Input: part model. Units: mm. Frame: model coordinates. Face numbers are marked on the shaded views. Coordinates: 2 decimals unless noted, no trailing zeros. Loops run counter-clockwise (first coordinate to the right, second up) from the corner with the lowest first, then second, coordinate; pieces in that order, holes last. Notation, with made-up numbers: M 30.5,72 L 65.5,72 A29 cw 65.5,95 Z; hole C -24.5,64 d3. An arc over 180 degrees is marked long. Use a Markdown table: item, result. Add a question column.
1. Draft query along Y for the marked faces 1 and 2. Return one class per face: +Y half, -Y half, draft (parallel to the pull), parting line (faces both ways), or undercut.
2. Line query: L1, parallel to X at y = 10, z = 0; L2, parallel to X at y = 9, z = 179; L3, parallel to Z at x = -277, y = 6.5. Output: solid intervals per line, ascending. Write a range as [from, to].
3. Pin query (flat end, axial travel): pin 1 (12 mm diameter, centred on x = 104.5, y = 2.5, fed in from +Z); pin 2 (1 mm diameter, centred on y = 4.5, z = -58.5, fed in from +X); pin 3 (12 mm diameter, centred on x = -34.5, y = 6.5, fed in from +Z). Return the tip coordinate at first contact, or that it passes through.
4. Section A-A on x = 0. Output: boundary loops of the cut face in (y, z), then the cut area to 3 significant figures.
5. Section B-B on z = 0. Output: boundary loops of the cut face in (x, y), then the cut area to 3 significant figures.
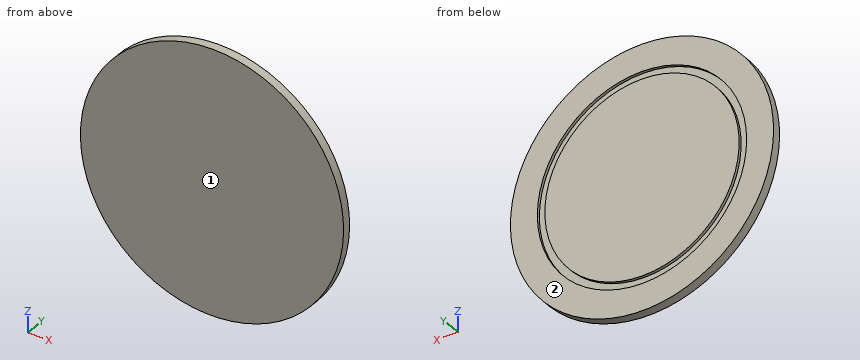
```python
from build123d import *

# Parameters (mm, degrees)
SKETCH1_R           = 440
BOSS_EXTRUDE1_DEPTH = 15
SKETCH2_R           = 350
SKETCH2_R_2         = 325
CUT_EXTRUDE1_DEPTH  = 10


with BuildPart() as part:
    # Sketch1 → Boss-Extrude1 (new, symmetric)
    with BuildSketch(Plane(origin=(0, 0, 0), x_dir=(1, 0, 0), z_dir=(0, 1, 0))):
        with Locations(Location((0, 0, 0), (0, 0, 270))):
            Circle(SKETCH1_R)
    extrude(amount=BOSS_EXTRUDE1_DEPTH, both=True)

    # Sketch2 → Cut-Extrude1 (cut)
    with BuildSketch(Plane(origin=(0, 15, 0), x_dir=(1, 0, 0), z_dir=(0, 1, 0))):
        with Locations(Location((0, 0, 0), (0, 0, 270))):
            Circle(SKETCH2_R)
        with Locations(Location((0, 0, 0), (0, 0, 270))):
            Circle(SKETCH2_R_2, mode=Mode.SUBTRACT)
    extrude(amount=-CUT_EXTRUDE1_DEPTH, mode=Mode.SUBTRACT)


solid = part.part
```
Answers below:
| question | item | result |
|---|---|---|
| 1 | face 1 | -Y half |
| 1 | face 2 | +Y half |
| 2 | L1 | x = [-440, -350], [-325, 325], [350, 440] |
| 2 | L2 | x = [-401.94, -300.76], [-271.26, 271.26], [300.76, 401.94] |
| 2 | L3 | z = [-341.86, -213.94], [-169.99, 169.99], [213.94, 341.86] |
| 3 | pin 1 | stops at z = 428.83 |
| 3 | pin 2 | stops at x = 436.16 |
| 3 | pin 3 | stops at z = 439.08 |
| 4 | outline | M -15,-440 L 15,-440 L 15,-350 L 5,-350 L 5,-325 L 15,-325 L 15,325 L 5,325 L 5,350 L 15,350 L 15,440 L -15,440 Z |
| 4 | area | 25,900 mm² |
| 5 | outline | M -440,-15 L 440,-15 L 440,15 L 350,15 L 350,5 L 325,5 L 325,15 L -325,15 L -325,5 L -350,5 L -350,15 L -440,15 Z |
| 5 | area | 25,900 mm² |
